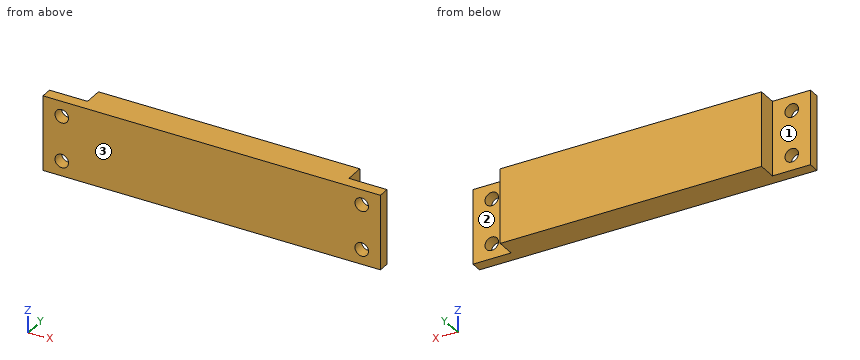
```python
from build123d import *

# Parameters (mm, degrees)
SKETCH1_W                = 10.15
SKETCH1_H                = 20
SKETCH1_W_2              = 69.7
BOSS_EXTRUDE1_DEPTH      = 3
SKETCH1_3_W              = 69.7
SKETCH1_3_H              = 20
BOSS_EXTRUDE2_DEPTH      = 8
M3_CLEARANCE_HOLE1_D     = 3.6
M3_CLEARANCE_HOLE1_DEPTH = 10
M3_CLEARANCE_HOLE1_TIP   = 1.081549114


with BuildPart() as part:
    # Sketch1 → Boss-Extrude1 (new body)
    with BuildSketch(Plane(origin=(0, 0, 0), x_dir=(1, 0, 0), z_dir=(0, 1, 0))):
        with Locations((-39.925, 0)):
            Rectangle(SKETCH1_W, SKETCH1_H)
        Rectangle(SKETCH1_W_2, SKETCH1_H)
        with Locations((39.925, 0)):
            Rectangle(SKETCH1_W, SKETCH1_H)
    extrude(amount=BOSS_EXTRUDE1_DEPTH)

    # Sketch1_3 → Boss-Extrude2 (add)
    with BuildSketch(Plane(origin=(0, 0, 0), x_dir=(1, 0, 0), z_dir=(0, 1, 0))):
        Rectangle(SKETCH1_3_W, SKETCH1_3_H)
    extrude(amount=BOSS_EXTRUDE2_DEPTH)

    # M3 Clearance Hole1
    with Locations(Plane(origin=(0, 3, 0), x_dir=(1, 0, 0), z_dir=(0, 1, 0))):
        with Locations((-40, 6), (-40, -6), (40, -6), (40, 6)):
            Hole(M3_CLEARANCE_HOLE1_D / 2, depth=M3_CLEARANCE_HOLE1_DEPTH)
            with Locations((0, 0, -(M3_CLEARANCE_HOLE1_DEPTH + M3_CLEARANCE_HOLE1_TIP / 2))):  # 118° drill point
                Cone(0, M3_CLEARANCE_HOLE1_D / 2, M3_CLEARANCE_HOLE1_TIP, mode=Mode.SUBTRACT)


solid = part.part
```
CAD build for the part. Positions are in the model's coordinates, mm. Face numbers are marked on the shaded views. A direction names the side the tool comes from. Give positions to 0.01 mm unless a question says otherwise; leave off trailing zeros. Order: outer loops, then holes, each group sorted by start corner. A loop starts at its lowest first (then second) coordinate and runs counter-clockwise, first axis right, second up.
(1) Saw through at A-A, the plane z = -6. Give the cut face in (x, y).
(2) Saw through at C-C, the plane x = -40. Give the cut face in (y, z), then the cut area to 3 significant figures.
(3) Saw through at D-D, the plane z = -1.5. Give the cut face in (x, y).
(4) Flat gauge pins, fed straight in: pin 1 (4 mm diameter, centred on y = 6, z = -3, fed in from +X); pin 2 (3 mm diameter, centred on x = 40, z = 6, fed in from -Y); pin 3 (1.5 mm diameter, centred on y = 4.5, z = -2.5, fed in from -X); pin 4 (8 mm diameter, centred on x = 41.5, z = 1.5, fed in from +Y). Where does each tip first touch, or does it go through?
(5) Drill centre lines: L1, parallel to X at y = 2.4, z = -6; L2, parallel to Z at x = -40, y = 1.3; L3, parallel to X at y = 6.75, z = 8.75. Where is each one in solid material? Low to high.
(6) Tool access for the marked faces 1, 2 and 3: list every direction of +Z, -Z, +X, -X, +Y, -Y with a clear straight run to the whole face (end or side of a thin tool).
(7) Saw through at B-B, the plane y = 1.5. Give the cut face in (x, z).
Results found:
1. outline: (-45, 0) - (-41.8, 0) - (-41.8, 3) - (-45, 3) - close; (-38.2, 0) - (38.2, 0) - (38.2, 3) - (34.85, 3) - (34.85, 8) - (-34.85, 8) - (-34.85, 3) - (-38.2, 3) - close; (41.8, 0) - (45, 0) - (45, 3) - (41.8, 3) - close
2. outline: (0, -10) - (3, -10) - (3, -7.8) - (0, -7.8) - close; (0, -4.2) - (3, -4.2) - (3, 4.2) - (0, 4.2) - close; (0, 7.8) - (3, 7.8) - (3, 10) - (0, 10) - close
2. area: 38.4 mm2
3. outline: (-45, 0) - (45, 0) - (45, 3) - (34.85, 3) - (34.85, 8) - (-34.85, 8) - (-34.85, 3) - (-45, 3) - close
4. pin 1: stops at x = 34.85
4. pin 2: passes through
4. pin 3: stops at x = -34.85
4. pin 4: stops at y = 3
5. L1: x = -45 to -41.8, -38.2 to 38.2, 41.8 to 45
5. L2: z = -10 to -7.8, -4.2 to 4.2, 7.8 to 10
5. L3: x = -34.85 to 34.85
6. face 1: +Z, -Z, -X, +Y
6. face 2: +Z, -Z, +X, +Y
6. face 3: +Z, -Z, +X, -X, -Y
7. outline: (-45, -10) - (45, -10) - (45, 10) - (-45, 10) - close; hole circle Ø3.6 at (-40, -6); hole circle Ø3.6 at (-40, 6); hole circle Ø3.6 at (40, -6); hole circle Ø3.6 at (40, 6)
